Autodesk Inventor part; units mm, degrees
ref_plane "YZ Plane" through (0, 0, 0) normal (1, 0, 0) x (0, 1, 0)
ref_plane "XZ Plane" through (0, 0, 0) normal (0, 1, 0) x (-1, 0, 0)
ref_plane "XY Plane" through (0, 0, 0) normal (0, 0, 1) x (1, 0, 0)
sketch "Sketch1" plane through (0, 0, 0) normal (0, 0, 1) x (1, 0, 0)
  circle A0 centre (0, 0) radius 20
  dimension "d0" = 40
extrude "Extrusion1" add sketch "Sketch1" along normal blind 6.6
sketch "Sketch3" plane through (0, 0, 0) normal (0, 0, -1) x (-1, 0, 0)
  circle A0 centre (0, 0) radius 17
  line L0 (0, 17) -> (0, 0)
  line L1 (0, 0) -> (14.7224, -8.5)
  line L2 (0, 0) -> (-14.7224, -8.5)
  line L3 (0, 0) -> (17, 0) construction
  line L4 (1.5, 16.9337) -> (1.5, 0.866)
  line L5 (-1.5, 16.9337) -> (-1.5, 0.866)
  line L6 (-1.5, 0.866) -> (-15.415, -7.1678)
  line L7 (0, -1.7321) -> (-13.915, -9.7659)
  line L8 (1.5, 0.866) -> (15.415, -7.1678)
  line L9 (0, -1.7321) -> (13.915, -9.7659)
  dimension "d6" = 34
  dimension "d7" = 120
  dimension "d8" = 150
  dimension "d9" = 1.5
  dimension "d10" = 1.5
  dimension "d11" = 1.5
  dimension "d12" = 1.5
  dimension "d13" = 1.5
  dimension "d14" = 1.5
extrude "Extrusion3" cut sketch "Sketch3" against normal up to surface (6.6 mm away) contours A0 L8 L4 | L5 L6 A0 | A0 L7 L9
sketch "Sketch5" plane through (0, 0, 6.6) normal (0, 0, 1) x (1, 0, 0)
  circle A0 centre (0, 0) radius 4
  dimension "d20" = 8
extrude "Extrusion5" add sketch "Sketch5" against normal blind 6.6
sketch "Sketch6" plane through (0, 0, 0) normal (0, 0, -1) x (-1, 0, 0)
  circle A0 centre (0, 0) radius 1.5
  line L0 (0, -1.5) -> (0, -4)
  arc A1 (-2.4613, -3.1531) -> (2.4613, -3.1531) centre (0, 0) ccw
  line L1 (0.5, -1.4142) -> (0.5, -3.9686)
  line L2 (-0.5, -1.4142) -> (-0.5, -3.9686)
  line L3 (-1.3266, 0.7) -> (1.3266, 0.7)
  point P0 (0.0845, 0.7)
  dimension "d23" = 3
  dimension "d24" = 0.5
  dimension "d25" = 0.5
  dimension "d29" = 2.2
extrude "Extrusion6" cut sketch "Sketch6" against normal up to surface (6.6 mm away) contours A0 L3 | L1 A1 L0 A0 | L0 A1 L2 A0 picked at (0, -0.0333)
fillet "Arredondamento1" radius 1 2 edges at (-20, 0, 6.6) (-20, 0, 0)
properties part number "wheel"
Here's how the part is built. I have some questions about the finished solid (model axes, mm). A direction names the side the tool comes from. Give positions to 0.01 mm unless a question says otherwise; leave off trailing zeros. Order: outer loops, then holes, each group sorted by start corner. A loop starts at its lowest first (then second) coordinate and runs counter-clockwise, first axis right, second up. Notation, with made-up numbers: M -5.75,39.25 L 12.25,39.25 A17 cw 12.25,54.25 Z; hole C -5,-11 d5. An arc over 180 degrees is marked long. Use a Markdown table: item, result. Add a question column.
1. Suppose I cut it at C-C (z = 3). List the corners of the cut face in (x, y) for me (3 decimals).
2. On a 3-axis mill with a long thin cutter (end or side, diameter ignored), from which of +Z, -Z, +X, -X, +Y, -Y can I reach the whole of each face in a straight line? I mean faces 1 (the cylindrical face through (-1.39, -0.56, 3.25)), 2 (the flat face through (0, 3, 0)). Say none if no direction works.
3. Suppose I cut it at B-B (y = 0). List the corners of the cut face in (x, z) for me, and give its area (3 significant figures).
4. Suppose I cut it at A-A (x = 0). List the corners of the cut face in (y, z) for me, and give its area (3 significant figures).
5. I need wall thicknesses on probe 1 along X at (y, z) = (-1.5, 2.25); probe 2 along Y at (x, z) = (11, 6); probe 3 along X at (y, z) = (5.5, 1.25). Which ranges of each line are inside material? Lowest first, please. Write a range as from..to.
6. For pin 1 Ø3 at (y, z) = (-3, 2.5) entering from -X; pin 2 Ø2 at (y, z) = (-2, 2.5) entering from +X (3 decimals); pin 3 Ø2 at (x, z) = (-5.5, 5) entering from +Y, each with a flat end and sliding along its axis, tell me the tip position at first contact or that it passes through.
7. If we mould it in two halves opening along X, with no side actions, what happens to faces 3 (the flat face through (0, 3, 6.6)), 4 (the cylindrical face through (1.52, -3.7, 3.35)), 5 (the cylindrical face through (-4.336, 19.524, 3.268))? For each: +X half, -X half, draft (parallel to the pull), parting line (faces both ways), or undercut.
8. Suppose I cut it at D-D (x = -8.5). Give the number of separate pieces and of enclosed holes in the cut face, and give its area (3 significant figures).
Results list:
| question | item | result |
|---|---|---|
| 1 | outline | C 0,0 d40; hole M -15.415,-7.168 L -3.961,-0.555 A4 cw -1.5,3.708 L -1.5,16.934 A17 ccw Z; hole M -13.915,-9.766 A17 ccw 13.915,-9.766 L 2.461,-3.153 A4 cw 0.5,-3.969 L 0.5,-1.414 A1.5 ccw 1.327,0.7 L -1.327,0.7 A1.5 ccw -0.5,-1.414 L -0.5,-3.969 A4 cw -2.461,-3.153 Z; hole M 1.5,3.708 A4 cw 3.961,-0.555 L 15.415,-7.168 A17 ccw 1.5,16.934 Z |
| 2 | face 1 | +Z, -Z |
| 2 | face 2 | -Z, +X, -X, +Y, -Y |
| 3 | outline | M -20,1 A1 ccw -19,0 L -17,0 L -17,6.6 L -19,6.6 A1 ccw -20,5.6 Z; M -4,0 L -1.5,0 L -1.5,6.6 L -4,6.6 Z; M 1.5,0 L 4,0 L 4,6.6 L 1.5,6.6 Z; M 17,0 L 19,0 A1 ccw 20,1 L 20,5.6 A1 ccw 19,6.6 L 17,6.6 Z |
| 3 | area | 71.7 mm² |
| 4 | outline | M -20,1 A1 ccw -19,0 L -17,0 L -17,6.6 L -19,6.6 A1 ccw -20,5.6 Z; M 0.7,0 L 19,0 A1 ccw 20,1 L 20,5.6 A1 ccw 19,6.6 L 0.7,6.6 Z |
| 4 | area | 146 mm² |
| 5 | probe 1 | x = -19.94..-16.93, -5.6..-0.5, 0.5..5.6, 16.93..19.94 |
| 5 | probe 2 | y = -16.6..-12.96, -8.08..-4.62, 12.96..16.6 |
| 5 | probe 3 | x = -19.23..-16.09, -1.5..1.5, 16.09..19.23 |
| 6 | pin 1 | stops at x = -19.94 |
| 6 | pin 2 | stops at x = 19.975 |
| 6 | pin 3 | stops at y = 19.49 |
| 7 | face 3 | draft |
| 7 | face 4 | undercut |
| 7 | face 5 | parting line |
| 8 | separate pieces | 3 |
| 8 | enclosed holes | 0 |
| 8 | area | 66.5 mm² |
